Work out the finished part from the listing and answer in its coordinate system (mm). Face numbers are marked on the shaded views. Give positions to 0.01 mm unless a question says otherwise; leave off trailing zeros. Loops run counter-clockwise (first coordinate to the right, second up) from the corner with the lowest first, then second, coordinate; pieces in that order, holes last. Notation, with made-up numbers: M -23,59.25 L -5,59.25 A12 ccw -5,63.25 Z; hole C 82,30.25 d1. An arc over 180 degrees is marked long. Answer in a Markdown table with one row per item. Add a question column.
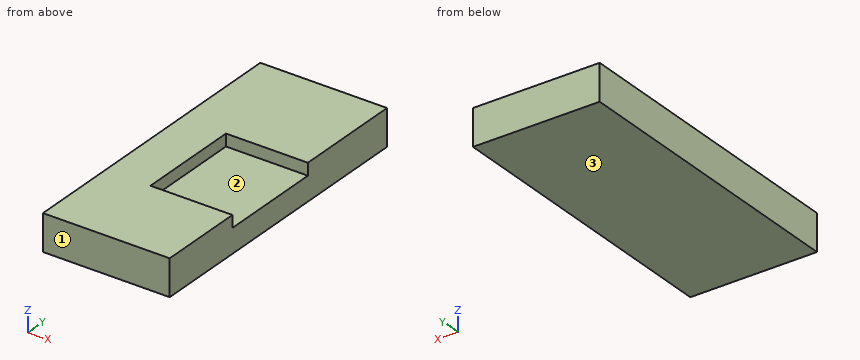
from build123d import *

# Parameters (mm, degrees)
F0_W     = 53.0420094728
F0_H     = 126.6452521086
F1_DEPTH = 10.16
F2_W     = 34.2897039372
F2_H     = 36.5310497582
F2_H_2   = 46.119553037
F3_DEPTH = 5.08


with BuildPart() as f1:
    # F0 (on Top) → F1 (new body)
    with BuildSketch(Plane.XY):
        with Locations((4.1718427092, -7.1517303586)):
            Rectangle(F0_W, F0_H)
    extrude(amount=F1_DEPTH)

    # F2 (on face) → F3 (join)
    with BuildSketch(Plane.XY.offset(10.16)):
        with Locations((13.547995477, -52.2088315338)):
            Rectangle(F2_W, F2_H)
        Polygon((-22.3491620272, 56.1708956957), (-22.3491620272, -70.4743564129), (-3.5968564916, -70.4743564129), (-3.5968564916, -33.9433066547), (-3.5968564916, 10.0513426587), (-3.5968564916, 56.1708956957), align=None)
        with Locations((13.547995477, 33.1111191772)):
            Rectangle(F2_W, F2_H_2)
    extrude(amount=F3_DEPTH)


solid = f1.part
(1) Each of these flat-tipped pins is pushed along its axis until it touches: P1, Ø5, axis at x = 14, y = -27.5, coming from the +Z side; P2, Ø2.5, axis at y = -2.5, z = 14, coming from the +X side. Where does it stop, or does it pass through?
(2) The mould has two halves that part along Y. Classify the marked faces 1, 2 and 3: pulls with the +Y half, pulls with the -Y half, needs draft (parallel to the pull), parting line crosses it, or undercut.
(3) Section B-B, the plane z = 12 is taken. Determine the outline of the cut face in (x, y).
(4) Consider line 1 along Y through (x, z) = (12, 10.5); line 2 along Z through (x, y) = (19.5, -9.5). Determine where each line is inside the solid, lowest interval first. Write a range as from..to.
(5) Section A-A, the plane x = 18 is taken. Determine the outline of the cut face in (y, z).
(6) Section C-C, the plane y = 6.5 is taken. Determine the outline of the cut face in (x, z), and give its area (3 significant figures).
Numbers:
| question | item | result |
|---|---|---|
| 1 | P1 | stops at z = 10.16 |
| 1 | P2 | stops at x = -3.6 |
| 2 | face 1 | pulls with the -Y half |
| 2 | face 2 | undercut |
| 2 | face 3 | needs draft |
| 3 | outline | M -22.35,-70.47 L 30.69,-70.47 L 30.69,-33.94 L -3.6,-33.94 L -3.6,10.05 L 30.69,10.05 L 30.69,56.17 L -22.35,56.17 Z |
| 4 | line 1 | y = -70.47..-33.94, 10.05..56.17 |
| 4 | line 2 | z = 0..10.16 |
| 5 | outline | M -70.47,0 L 56.17,0 L 56.17,15.24 L 10.05,15.24 L 10.05,10.16 L -33.94,10.16 L -33.94,15.24 L -70.47,15.24 Z |
| 6 | outline | M -22.35,0 L 30.69,0 L 30.69,10.16 L -3.6,10.16 L -3.6,15.24 L -22.35,15.24 Z |
| 6 | area | 634 mm² |
